CAD build for the part. Positions are in the model's coordinates, mm. Face numbers are marked on the shaded views. Coordinates: 2 decimals unless noted, no trailing zeros. Order: outer loops, then holes, each group sorted by start corner. A loop starts at its lowest first (then second) coordinate and runs counter-clockwise, first axis right, second up. Notation, with made-up numbers: (-20.5, 21) - (-3.5, 21) arc R11 ccw to (-3.5, 41) - close; hole circle Ø2 at (55.5, 32.25). An arc over 180 degrees is marked (long way). Write each question's results on one line, items separated by ' | '. Start each with the question number.
Q1. Band-saw the part on A-A, the plane z = 0. Write the cut outline in (x, y), then the cut area to 3 significant figures.
Q2. Band-saw the part on D-D, the plane z = -6.5. Write the cut outline in (x, y).
Q3. Pin check, flat tips, straight feed: P1, Ø11.5, axis at x = 0, z = 0, coming from the +Y side; P2, Ø2, axis at x = -13, y = -3.5, coming from the -Z side; P3, Ø2, axis at y = -1.5, z = 11, coming from the -X side; P4, Ø2, axis at y = -3.5, z = -13, coming from the +X side. Stop position of each tip, or through.
Q4. Band-saw the part on C-C, the plane y = -2.4. Write the cut outline in (x, z).
Q5. Band-saw the part on B-B, the plane x = 0. Write the cut outline in (y, z), then the cut area to 3 significant figures.
Q6. Wall check: probe 1 along Z at (x, y) = (0, -3.5); probe 2 along Y at (x, z) = (-27, -6); probe 3 along Z at (x, y) = (0, -1.05). Give the ranges that are in metal, low to high.
Q7. Pull direction X, two halves, no side cores. Call the marked faces 1 and 2: released by +X, released by -X, zero draft, split by the parting line, or undercut.
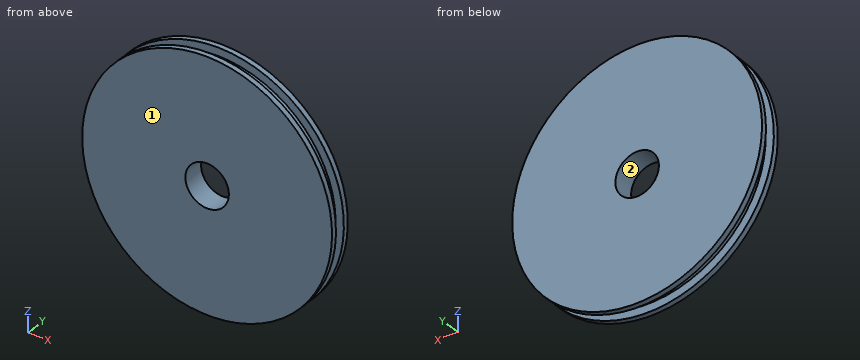
```python
from build123d import *

# Parameters (mm, degrees)
SKETCH6_R          = 5.0419
CUT_EXTRUDE1_DEPTH = 6.08


with BuildPart() as part:
    # Sketch1 → Revolve1 (revolve)
    with BuildSketch(Plane(origin=(0, 0, 0), x_dir=(0, 0, -1), z_dir=(1, 0, 0))):
        Polygon((0, 0), (0, -5.08), (-28.956, -5.08), (-28.956, -3.81), (-27.051, -3.81), (-27.051, -1.27), (-28.956, -1.27), (-28.956, 0), align=None)
    revolve(axis=Axis((0, 0, 0), (0, -1, 0)))

    # Sketch6 → Cut-Extrude1 (cut, through all)
    with BuildSketch(Plane.XZ.offset(5.08)):
        Circle(SKETCH6_R)
    extrude(amount=-CUT_EXTRUDE1_DEPTH, mode=Mode.SUBTRACT)


solid = part.part
```
Results below:
1) outline: (-28.96, -5.08) - (-5.04, -5.08) - (-5.04, 0) - (-28.96, 0) - (-28.96, -1.27) - (-27.05, -1.27) - (-27.05, -3.81) - (-28.96, -3.81) - close; (5.04, -5.08) - (28.96, -5.08) - (28.96, -3.81) - (27.05, -3.81) - (27.05, -1.27) - (28.96, -1.27) - (28.96, 0) - (5.04, 0) - close | area: 233 mm²
2) outline: (-28.22, -5.08) - (28.22, -5.08) - (28.22, -3.81) - (26.26, -3.81) - (26.26, -1.27) - (28.22, -1.27) - (28.22, 0) - (-28.22, 0) - (-28.22, -1.27) - (-26.26, -1.27) - (-26.26, -3.81) - (-28.22, -3.81) - close
3) P1: stops at y = 0 | P2: stops at z = -26.33 | P3: stops at x = -27.16 | P4: stops at x = 26.33
4) outline: circle Ø54.1 at (0, 0); hole circle Ø10.08 at (0, 0)
5) outline: (-5.08, -28.96) - (-3.81, -28.96) - (-3.81, -27.05) - (-1.27, -27.05) - (-1.27, -28.96) - (0, -28.96) - (0, -5.04) - (-5.08, -5.04) - close; (-5.08, 5.04) - (0, 5.04) - (0, 28.96) - (-1.27, 28.96) - (-1.27, 27.05) - (-3.81, 27.05) - (-3.81, 28.96) - (-5.08, 28.96) - close | area: 233 mm²
6) probe 1: z = -27.05 to -5.04, 5.04 to 27.05 | probe 2: y = -5.08 to -3.81, -1.27 to 0 | probe 3: z = -28.96 to -5.04, 5.04 to 28.96
7) face 1: zero draft | face 2: undercut
